Geometry: final body of the model. Coordinates: model frame, mm. Give positions to 0.01 mm unless a question says otherwise; leave off trailing zeros. Write each loop counter-clockwise with the first axis right and the second up, starting at its lowest first coordinate (ties: lowest second). Pieces come first, ordered by that corner, then holes. Notation, with made-up numbers: (-22, -30) - (15, -30) arc R19 ccw to (15, -26) - close; hole circle Ø2 at (54, 60). An arc over 180 degrees is marked (long way). Use CSV: the item, a comma, the result in double quotes. Start each with the question number.
(1) Section A-A on x = 7. Output: boundary loops of the cut face in (y, z), and give its area (4 significant figures).
(2) Section C-C on z = -7. Output: boundary loops of the cut face in (x, y), and give its area (4 significant figures).
(3) Section D-D on x = 60. Output: boundary loops of the cut face in (y, z), and give its area (3 significant figures).
(4) Draft query along Z for faces 1 (the cylindrical face through (6.512, 2.218, -120.804)), 2 (the flat face through (130, 2, -64)), 3 (the flat face through (64, 2, -130)). Return one class per face: released by +Z, released by -Z, zero draft, split by the parting line, or undercut.
(5) First-contact query: pin 1 Ø3.5 at (x, z) = (7, -123) entering from -Y. Flat tip, straight axial feed; report the tip coordinate or a pass-through.
(6) Section B-B on y = 2.35. Count the separate pieces of the cut face and the enclosed holes in it, and give its area (3 significant figures).
(7) Line query: probe 1 along X at (y, z) = (1.45, -29); probe 2 along Z at (x, y) = (65, 1.75); probe 3 along X at (y, z) = (3.05, -123). Output: solid intervals per line, ascending. Write a range as [from, to].
from build123d import *

# Parameters (mm, degrees)
SKETCH1_W           = 130
SKETCH1_H           = 130
SKETCH1_R           = 13.4
SKETCH1_R_2         = 2.25
BOSS_EXTRUDE1_DEPTH = 4.5
SKETCH2_R           = 0.25
CUT_EXTRUDE1_DEPTH  = 5.5


with BuildPart() as part:
    # Sketch1 → Boss-Extrude1 (new body)
    with BuildSketch(Plane(origin=(0, 0, 0), x_dir=(1, 0, 0), z_dir=(0, 1, 0))):
        with Locations((65, 65)):
            Rectangle(SKETCH1_W, SKETCH1_H)
        with Locations((65, 65)):
            Circle(SKETCH1_R, mode=Mode.SUBTRACT)
        with Locations((123, 123)):
            Circle(SKETCH1_R_2, mode=Mode.SUBTRACT)
        with Locations((123, 7)):
            Circle(SKETCH1_R_2, mode=Mode.SUBTRACT)
        with Locations((7, 7)):
            Circle(SKETCH1_R_2, mode=Mode.SUBTRACT)
        with Locations((7, 123)):
            Circle(SKETCH1_R_2, mode=Mode.SUBTRACT)
    extrude(amount=BOSS_EXTRUDE1_DEPTH)

    # Sketch2 → Cut-Extrude1 (cut, through all)
    with BuildSketch(Plane.XZ):
        with Locations((29, -65)):
            Circle(SKETCH2_R)
        with Locations((65, -29)):
            Circle(SKETCH2_R)
        with Locations((101, -65)):
            Circle(SKETCH2_R)
        with Locations((65, -101)):
            Circle(SKETCH2_R)
        with Locations((101, -29)):
            Circle(SKETCH2_R)
        with Locations((29, -29)):
            Circle(SKETCH2_R)
        with Locations((101, -101)):
            Circle(SKETCH2_R)
        with Locations((29, -101)):
            Circle(SKETCH2_R)
    extrude(amount=-CUT_EXTRUDE1_DEPTH, mode=Mode.SUBTRACT)


solid = part.part
Check values:
1,outline,"(0, -130) - (4.5, -130) - (4.5, -125.25) - (0, -125.25) - close; (0, -120.75) - (4.5, -120.75) - (4.5, -9.25) - (0, -9.25) - close; (0, -4.75) - (4.5, -4.75) - (4.5, 0) - (0, 0) - close"
1,area,"544.5 mm²"
2,outline,"(0, 0) - (4.75, 0) - (4.75, 4.5) - (0, 4.5) - close; (9.25, 0) - (120.75, 0) - (120.75, 4.5) - (9.25, 4.5) - close; (125.25, 0) - (130, 0) - (130, 4.5) - (125.25, 4.5) - close"
2,area,"544.5 mm²"
3,outline,"(0, -130) - (4.5, -130) - (4.5, -77.43) - (0, -77.43) - close; (0, -52.57) - (4.5, -52.57) - (4.5, 0) - (0, 0) - close"
3,area,"473 mm²"
4,face 1,"undercut"
4,face 2,"zero draft"
4,face 3,"released by -Z"
5,pin 1,"passes through"
6,separate pieces,"1"
6,enclosed holes,"13"
6,area,"16,300 mm²"
7,probe 1,"x = [0, 28.75], [29.25, 64.75], [65.25, 100.75], [101.25, 130]"
7,probe 2,"z = [-130, -101.25], [-100.75, -78.4], [-51.6, -29.25], [-28.75, 0]"
7,probe 3,"x = [0, 4.75], [9.25, 120.75], [125.25, 130]"
